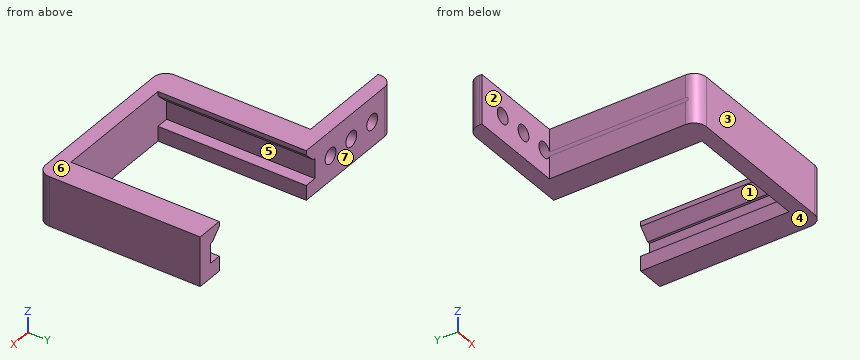
from build123d import *

# Parameters (mm, degrees)
F1_DEPTH    = 20
F3_D        = 6.2484
F4_W        = 60
F4_H        = 6
F6_DEPTH    = 5
F5_W        = 60
F5_H        = 5.8524994925
F5_H_2      = 5.9575000778
F7_DEPTH    = 5
F8_SIZE     = 4
F9_T1_DEPTH = 45
F9_T3_DEPTH = 34.127861456
F9_T5_DEPTH = 34.127861456


# Not quite as in the source:
# - a fillet or chamfer that OpenCascade refuses, or shapes differently, is made with other operations: its cross-section is extruded or revolved along the edge and cut away or added


with BuildPart() as f1:
    # F0 (on Top) → F1 (new body)
    with BuildSketch(Plane.XY):
        Polygon((45, 0), (0, 0), (0, -6), (39, -6), (39, -66), (111.2, -66), (111.2, 0), (105.2, 0), (105.2, -60), (45, -60), align=None)
    extrude(amount=F1_DEPTH)

    # F3 (through all)
    with Locations(Plane(origin=(0, 0, 0), x_dir=(-1, 0, 0), z_dir=(0, 1, 0))):
        with Locations((-36, 10), (-24, 10), (-12, 10)):
            Hole(F3_D / 2)

    # F4 (on face) → F6 (join)
    with BuildSketch(Plane(origin=(105.2, 0, 0), x_dir=(0, -1, 0), z_dir=(-1, 0, 0))):
        with Locations((30, 17)):
            Rectangle(F4_W, F4_H)
        with Locations((30, 3)):
            Rectangle(F4_W, F4_H)
    extrude(amount=F6_DEPTH)

    # F5 (on face) → F7 (join)
    with BuildSketch(Plane.YZ.offset(45)):
        with Locations((-30, 17.0737502538)):
            Rectangle(F5_W, F5_H)
        with Locations((-30, 2.9787500389)):
            Rectangle(F5_W, F5_H_2)
    extrude(amount=F7_DEPTH)

    # F8
    f8_edges = [f1.edges().sort_by_distance(p)[0] for p in [
        (50, -30, 14.147501),
        (100.2, -30, 14),
    ]]
    chamfer(f8_edges, length=F8_SIZE)

    # F9: fillet of radius 5 on 4 edges, made by hand

    # F9_s2 → F9_t1 (cut)
    with BuildSketch(Plane.XY.offset(-12.5)):
        with BuildLine():
            ThreePointArc((106.2, -66), (109.7355339059, -64.5355339059), (111.2, -61))
            Line((111.2, -61), (111.2, -66))
            Line((111.2, -66), (106.2, -66))
        make_face()
        with BuildLine():
            ThreePointArc((5, 0), (1.4644660941, -1.4644660941), (0, -5))
            Line((0, -5), (0, 0))
            Line((0, 0), (5, 0))
        make_face()
    extrude(amount=F9_T1_DEPTH, mode=Mode.SUBTRACT)

    # F9_s4 → F9_t3 (cut)
    with BuildSketch(Plane.XY.offset(-1.627861456)):
        with BuildLine():
            ThreePointArc((39, -61), (40.4644660941, -64.5355339059), (44, -66))
            Line((44, -66), (39, -66))
            Line((39, -66), (39, -61))
        make_face()
    extrude(amount=F9_T3_DEPTH, mode=Mode.SUBTRACT)

    # F9_s6 → F9_t5 (cut)
    with BuildSketch(Plane.XY.offset(-12.5)):
        with BuildLine():
            ThreePointArc((44, -66), (40.4644660941, -64.5355339059), (39, -61))
            Line((39, -61), (39, -66))
            Line((39, -66), (44, -66))
        make_face()
    extrude(amount=F9_T5_DEPTH, mode=Mode.SUBTRACT)


solid = f1.part
The listing builds one solid part. Answer for the finished solid, in the listing's coordinates (mm). Face numbers are marked on the shaded views. A direction names the side the tool comes from. Coordinates: 2 decimals unless noted, no trailing zeros. Order: outer loops, then holes, each group sorted by start corner. A loop starts at its lowest first (then second) coordinate and runs counter-clockwise, first axis right, second up.
Q1. A cutting plane is placed at B-B, the plane x = 24. Write down the section's boundary in (y, z).
Q2. A cutting plane is placed at A-A, the plane y = -21.5. Write down the section's boundary in (x, z).
Q3. Given P1, Ø6.5, axis at y = -33.5, z = 11, coming from the -X side; P2, Ø5, axis at x = 100, y = -18.5, coming from the -Z side; P3, Ø5, axis at x = 24, z = 10, coming from the +Y side; P4, Ø3, axis at x = 57, z = 17, coming from the +Y side, each flat-ended and moving along its own axis, determine where each tip first touches the part or whether it passes through.
Q4. Consider line 1 (X direction, y = -15.5, z = 12.75); line 2 (Z direction, x = 24, y = -3); line 3 (Z direction, x = 47, y = -7). Determine where each line is inside the solid, lowest interval first.
Q5. A cutting plane is placed at C-C, the plane z = 16. Write down the section's boundary in (x, y), and give its area (3 significant figures).
Q6. A cutting plane is placed at D-D, the plane x = 80. Write down the section's boundary in (y, z), and give its area (3 significant figures).
Q7. Which of the six approach directions +Z, -Z, +X, -X, +Y, -Y give full straight-line access (tool end or side, diameter ignored) to the marked faces 1, 2 and 3?
Q8. For a pull along Z with two mould halves and no side action, classify the marked faces 4, 5, 6 and 7 as pulls with the +Z half, pulls with the -Z half, needs draft (parallel to the pull), parting line crosses it, or undercut.
Answers follow:
1. outline: (-6, 0) - (0, 0) - (0, 6.88) - (-6, 6.88) - close; (-6, 13.12) - (0, 13.12) - (0, 20) - (-6, 20) - close
2. outline: (39, 0) - (50, 0) - (50, 5.96) - (45, 5.96) - (45, 14.15) - (46, 14.15) - (50, 18.15) - (50, 20) - (39, 20) - (39, 10.87) arc R3.12 cw to (39, 9.13) - close; (100.2, 0) - (111.2, 0) - (111.2, 20) - (100.2, 20) - (100.2, 18) - (104.2, 14) - (105.2, 14) - (105.2, 6) - (100.2, 6) - close
3. P1: stops at x = 39
3. P2: stops at z = 0
3. P3: passes through
3. P4: stops at y = -60
4. line 1: x = 39 to 45, 105.2 to 111.2
4. line 2: z = 0 to 6.88, 13.12 to 20
4. line 3: z = 0 to 5.96, 15.15 to 20
5. outline: (0, -6) - (39, -6) - (39, -61) arc R5 ccw to (44, -66) - (106.2, -66) arc R5 ccw to (111.2, -61) - (111.2, 0) - (102.2, 0) - (102.2, -60) - (47.85, -60) - (47.85, 0) - (5, 0) arc R5 ccw to (0, -5) - close
5. area: 1,720 mm2
6. outline: (-66, 0) - (-60, 0) - (-60, 20) - (-66, 20) - close
6. area: 120 mm2
7. face 1: +Y
7. face 2: +Z, -Z, -X, -Y
7. face 3: +Z, -Z, +X, -X, -Y
8. face 4: pulls with the -Z half
8. face 5: undercut
8. face 6: pulls with the +Z half
8. face 7: needs draft
